from build123d import *

# Parameters (mm, degrees)
SKETCH4_R          = 15
CUT_EXTRUDE1_DEPTH = 15


with BuildPart() as part:
    # Sketch1 → Revolve1 (revolve)
    with BuildSketch(Plane.XY):
        with BuildLine():
            Line((0, 22.5), (0, -22.5))
            ThreePointArc((0, -22.5), (22.5, 0), (0, 22.5))
        make_face()
    revolve(axis=Axis((0, 22.5, 0), (0, -1, 0)))

    # Sketch2 → Cut-Revolve6 (revolve, cut)
    with BuildSketch(Plane.XY):
        with BuildLine():
            Line((5, 19.917809385), (-5, 19.917809385))
            Line((-5, 19.917809385), (-5, 21.917809385))
            ThreePointArc((-5, 21.917809385), (0, 22.480888956), (5, 21.917809385))
            Line((5, 21.917809385), (5, 19.917809385))
        make_face()
    revolve(axis=Axis((0, 0, 0), (-1, 0, 0)), mode=Mode.SUBTRACT)

    # Sketch4 → Cut-Extrude1 (cut)
    with BuildSketch(Plane(origin=(22.5, 0, 0), x_dir=(0, 0, -1), z_dir=(1, 0, 0))):
        Circle(SKETCH4_R)
    extrude(amount=-CUT_EXTRUDE1_DEPTH, mode=Mode.SUBTRACT)


solid = part.part
Can you work these out from the model? Positions are in its coordinate system, mm. A direction names the side the tool comes from. Give positions to 0.01 mm unless a question says otherwise; leave off trailing zeros. Loops run counter-clockwise (first coordinate to the right, second up) from the corner with the lowest first, then second, coordinate; pieces in that order, holes last. Notation, with made-up numbers: (45.5, 41.25) -> (82.5, 41.25) arc R17 cw to (82.5, 59.25) -> close; hole circle Ø5 at (85, 47.25). An arc over 180 degrees is marked (long way). Return JSON: item names as keys, results as strings.
Q1. On a 3-axis mill with a long thin cutter (end or side, diameter ignored), from which of +Z, -Z, +X, -X, +Y, -Y can I reach the whole of each face in a straight line? I mean faces 1 (the face through (12.2, 0.66, 14.985)), 2 (the face through (-0.07, -14.68, -13.46)). Say none if no direction works.
Checks:
{"face 1": "+X", "face 2": "none"}
Q2. I want a section at C-C, the plane x = 9. List the corners of the cut face in (y, z) for me, then the cut area to 3 significant figures.
Checks:
{"outline": "circle Ø41.24 at (0, 0); hole circle Ø30 at (0, 0)", "area": "629 mm2"}
Q3. For pin 1 Ø8 at (y, z) = (2.5, 8) entering from +X; pin 2 Ø2 at (x, y) = (12, -17) entering from -Z; pin 3 Ø2 at (y, z) = (4, 7.5) entering from -X; pin 4 Ø8 at (y, z) = (-0.5, 12.5) entering from +X, each with a flat end and sliding along its axis, tell me the tip position at first contact or that it passes through.
Checks:
{"pin 1": "stops at x = 7.5", "pin 2": "stops at z = -10.67", "pin 3": "stops at x = -21.21", "pin 4": "stops at x = 16.77"}
Q4. I want a section at D-D, the plane x = -11.5. List the corners of the cut face in (y, z) for me.
Checks:
{"outline": "circle Ø38.68 at (0, 0)"}
Q5. I want a section at A-A, the plane z = 0. List the corners of the cut face in (x, y) for me.
Checks:
{"outline": "(7.5, -15) -> (7.5, 15) -> (16.77, 15) arc R22.5 ccw (long way) to (16.77, -15) -> close; hole (-5, -21.92) arc R22.48 ccw to (5, -21.92) -> (5, -19.92) -> (-5, -19.92) -> close; hole (-5, 19.92) -> (5, 19.92) -> (5, 21.92) arc R22.48 ccw to (-5, 21.92) -> close"}
Q6. I need wall thicknesses on probe 1 along Z at (x, y) = (12.25, 0); probe 2 along X at (y, z) = (-1, 0); probe 3 along Z at (x, y) = (14, 4.5). Which ranges of each line are inside material? Lowest first, please.
Checks:
{"probe 1": "z = -18.87 to -15, 15 to 18.87", "probe 2": "x = -22.48 to 7.5", "probe 3": "z = -17.03 to -14.31, 14.31 to 17.03"}
Q7. We'd pull the mould along X, two halves only. Please class faces 3 (the face through (7.5, 0, 0)), 4 (the face through (-5, -10, 18)): released by +X, released by -X, zero draft, split by the parting line, or undercut.
Checks:
{"face 3": "released by +X", "face 4": "undercut"}
